```python
from build123d import *

# Parameters (mm, degrees)
ESTRUSIONE_ESTRUSIONE1_DEPTH = 17
SCHIZZO4_W                   = 11
SCHIZZO4_H                   = 17
TAGLIO_ESTRUSIONE3_DEPTH     = 17
RACCORDO3_START              = -1
RACCORDO3_DEPTH              = 19
TAGLIO_ESTRUSIONE4_DEPTH     = 32.272991542
TAGLIO_ESTRUSIONE5_DEPTH     = 32.272991542


with BuildPart() as part:
    # Schizzo1 → Estrusione-Estrusione1 (new body)
    with BuildSketch(Plane(origin=(0, 0, 0), x_dir=(0, 0, -1), z_dir=(1, 0, 0))):
        with BuildLine():
            Line((0, 19.5), (0, 0.5))
            ThreePointArc((0, 0.5), (0.146446609, 0.146446609), (0.5, 0))
            Line((0.5, 0), (19.5, 0))
            ThreePointArc((19.5, 0), (19.853553391, 0.146446609), (20, 0.5))
            Line((20, 0.5), (20, 3))
            Line((20, 3), (3, 20))
            Line((3, 20), (0.5, 20))
            ThreePointArc((0.5, 20), (0.146446609, 19.853553391), (0, 19.5))
        make_face()
    extrude(amount=ESTRUSIONE_ESTRUSIONE1_DEPTH)

    # Schizzo4 → Taglio-Estrusione3 (cut)
    with BuildSketch(Plane(origin=(0, 0, -20), x_dir=(-1, 0, 0), z_dir=(0, 0, -1))):
        with Locations((-8.5, 11.5)):
            Rectangle(SCHIZZO4_W, SCHIZZO4_H)
    extrude(amount=-TAGLIO_ESTRUSIONE3_DEPTH, mode=Mode.SUBTRACT)

    # Raccordo3: read off the stored shape, not the designer's step
    # Raccordo3 outline → Raccordo3 (cut)
    with BuildSketch(Plane.YZ.offset(RACCORDO3_START)):
        with BuildLine():
            Line((3, -20), (3.146446609, -19.853553391))
            ThreePointArc((3.146446609, -19.853553391), (2.984234935, -19.961939766), (2.792893219, -20))
            Line((2.792893219, -20), (3, -20))
        make_face()
        with BuildLine():
            Line((19.853553391, -3.146446609), (20, -3))
            Line((20, -3), (20, -2.792893219))
            ThreePointArc((20, -2.792893219), (19.961939766, -2.984234935), (19.853553391, -3.146446609))
        make_face()
    extrude(amount=RACCORDO3_DEPTH, mode=Mode.SUBTRACT)

    # Schizzo5 → Taglio-Estrusione4 (cut, through all)
    with BuildSketch(Plane(origin=(0, 3, 0), x_dir=(1, 0, 0), z_dir=(0, 1, 0))):
        with BuildLine():
            Line((11.5, 11.455089861), (11.5, 8.455089861))
            ThreePointArc((11.5, 8.455089861), (8.5, 5.455089861), (5.5, 8.455089861))
            Line((5.5, 8.455089861), (5.5, 11.455089861))
            ThreePointArc((5.5, 11.455089861), (8.5, 14.455089861), (11.5, 11.455089861))
        make_face()
    extrude(amount=-TAGLIO_ESTRUSIONE4_DEPTH, mode=Mode.SUBTRACT)

    # Schizzo6 → Taglio-Estrusione5 (cut, through all)
    with BuildSketch(Plane(origin=(0, 0, -3), x_dir=(-1, 0, 0), z_dir=(0, 0, -1))):
        with BuildLine():
            Line((-5.5, 11.455089861), (-5.5, 8.455089861))
            ThreePointArc((-5.5, 8.455089861), (-8.5, 5.455089861), (-11.5, 8.455089861))
            Line((-11.5, 8.455089861), (-11.5, 11.455089861))
            ThreePointArc((-11.5, 11.455089861), (-8.5, 14.455089861), (-5.5, 11.455089861))
        make_face()
    extrude(amount=-TAGLIO_ESTRUSIONE5_DEPTH, mode=Mode.SUBTRACT)


solid = part.part
```
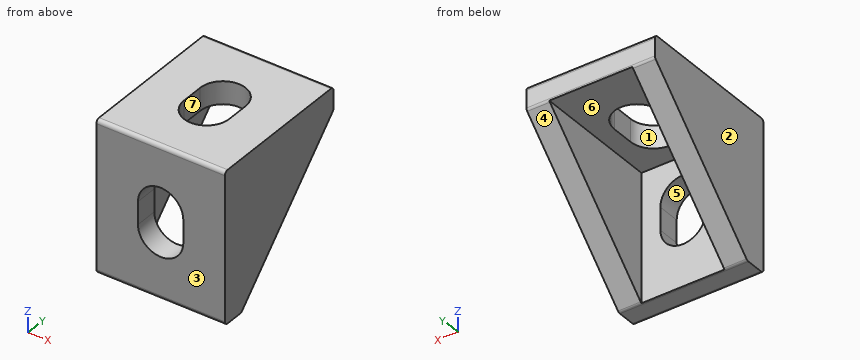
For this review, take the finished solid that the model builds, in its own axes (mm). Face numbers are marked on the shaded views. A direction names the side the tool comes from. Round coordinates to 2 decimals unless told otherwise and drop trailing zeros. Write each loop counter-clockwise with the first axis right and the second up, starting at its lowest first coordinate (ties: lowest second). Pieces come first, ordered by that corner, then holes. Notation, with made-up numbers: (77.5, -18.75) -> (108.5, -18.75) arc R9 cw to (108.5, -12.75) -> close; hole circle Ø8 at (-33, -16.5). An arc over 180 degrees is marked (long way). One line per question, with ' | ' between items. Start each with the question number.
(1) Add section B-B, the plane y = 10. Write out the cut boundary in (x, z).
(2) Tool access review of the marked faces 5, 6 and 7: name each direction out of +Z, -Z, +X, -X, +Y, -Y from which nothing blocks a thin tool from reaching the whole face with its end or side.
(3) Add section D-D, the plane x = 15. Write out the cut boundary in (y, z), plus the area to 3 significant figures.
(4) Add section A-A, the plane x = 8.5. Write out the cut boundary in (y, z), plus the area to 3 significant figures.
(5) For line 1 along X through (y, z) = (4.25, -9); line 2 along Z through (x, y) = (13.5, 8.75); line 3 along Y through (x, z) = (12.75, -10), list the stretches that pass through material, from the lowest coordinate up. Write a range as from..to.
(6) Insertion check: P1, Ø4, axis at x = 9.5, z = -15, coming from the +Y side; P2, Ø5.5, axis at x = 7, y = 9, coming from the -Z side. Each pin has a flat end and moves straight along its axis. Give the tip position at first contact, or say it passes through.
(7) Mouldability with a two-part tool opening along Y and no side actions: class the marked faces 1, 2, 3 and 4 as released by +Y, released by -Y, zero draft, split by the parting line, or undercut.
(8) Add section C-C, the plane z = -6. Write out the cut boundary in (x, y).
Answer list:
1) outline: (0, -13) -> (3, -13) -> (3, -3) -> (5.5, -3) -> (5.5, 0) -> (0, 0) -> close; (11.5, -3) -> (14, -3) -> (14, -13) -> (17, -13) -> (17, 0) -> (11.5, 0) -> close
2) face 5: +Y, -Y | face 6: -Z, +Y | face 7: +Z, -Z
3) outline: (0, -19.5) arc R0.5 ccw to (0.5, -20) -> (2.79, -20) arc R0.5 ccw to (3.15, -19.85) -> (19.85, -3.15) arc R0.5 ccw to (20, -2.79) -> (20, -0.5) arc R0.5 ccw to (19.5, 0) -> (0.5, 0) arc R0.5 ccw to (0, -0.5) -> close | area: 255 mm²
4) outline: (0, -19.5) arc R0.5 ccw to (0.5, -20) -> (2.79, -20) arc R0.5 ccw to (3, -19.96) -> (3, -14.46) -> (0, -14.46) -> close; (0, -5.46) -> (3, -5.46) -> (3, -3) -> (5.46, -3) -> (5.46, 0) -> (0.5, 0) arc R0.5 ccw to (0, -0.5) -> close; (14.46, -3) -> (19.96, -3) arc R0.5 ccw to (20, -2.79) -> (20, -0.5) arc R0.5 ccw to (19.5, 0) -> (14.46, 0) -> close | area: 56.8 mm²
5) line 1: 0..3, 14..17 | line 2: -3..0 | line 3: 0..3
6) P1: y = 3 | P2: z = -3
7) face 1: undercut | face 2: zero draft | face 3: released by -Y | face 4: released by +Y
8) outline: (0, 0) -> (6.78, 0) -> (6.78, 3) -> (3, 3) -> (3, 17) -> (0, 17) -> close; (10.22, 0) -> (17, 0) -> (17, 17) -> (14, 17) -> (14, 3) -> (10.22, 3) -> close
